The listing builds one solid part. Answer for the finished solid, in the listing's coordinates (mm). Face numbers are marked on the shaded views. A direction names the side the tool comes from. Round coordinates to 2 decimals unless told otherwise and drop trailing zeros. Write each loop counter-clockwise with the first axis right and the second up, starting at its lowest first coordinate (ties: lowest second). Pieces come first, ordered by that corner, then holes.
Item 1: Find the intervals of material crossed by probe 1 along Z at (x, y) = (0, 0.2); probe 2 along Y at (x, z) = (3, -3.5); probe 3 along Y at (x, z) = (2.75, -5), in increasing order.
Item 2: Find section A-A on x = 0. Give the vertices of the cut face in (y, z).
Item 3: A tool of negligible diameter and unlimited length cuts with its end or side. For the marked faces 4, 5 and 6, from which of +Z, -Z, +X, -X, +Y, -Y can it reach the whole face along a straight path? Write none if from no direction.
Item 4: For a pull along Z with two mould halves and no side action, classify the marked faces 1, 2 and 3 as +Z half, -Z half, draft (parallel to the pull), parting line (faces both ways), or undercut.
Item 5: Each of these flat-tipped pins is pushed along its axis until it touches: pin 1 (6 mm diameter, centred on x = -0.5, y = -9, fed in from +Z); pin 2 (3 mm diameter, centred on x = 3, y = -9, fed in from -Z). Where does it stop, or does it pass through?
Item 6: Find section C-C on y = -4.25. Give the vertices of the cut face in (x, z), then the cut area to 3 significant figures.
Item 7: Find section B-B on z = 2.75. Give the vertices of the cut face in (x, y).
```python
from build123d import *

# Parameters (mm, degrees)
EXTRUDE_1_DEPTH              = 3
SKETCH_2_R                   = 5
EXTRUDE_2_DEPTH              = 10
HOLE_WIZARD_M4_1_D           = 6
HOLE_WIZARD_M4_1_CBORE_D     = 10
HOLE_WIZARD_M4_1_CBORE_DEPTH = 4.5


with BuildPart() as part:
    # 草图1 → 凸台-拉伸1 (new, symmetric)
    with BuildSketch(Plane(origin=(0, 0, 0), x_dir=(1, 0, 0), z_dir=(0, 1, 0))):
        Polygon((6.92820323, 0), (3.464101615, 6), (-3.464101615, 6), (-6.92820323, 0), (-3.464101615, -6), (3.464101615, -6), align=None)
    extrude(amount=EXTRUDE_1_DEPTH, both=True)

    # 草图2 → 凸台-拉伸2 (add)
    with BuildSketch(Plane.XZ.offset(3)):
        with Locations(Location((0, 0, 0), (0, 0, 90))):
            Circle(SKETCH_2_R)
    extrude(amount=EXTRUDE_2_DEPTH)

    # M4 六角头螺栓的柱形沉头孔1 (through all)
    with Locations(Plane(origin=(0, 3, 0), x_dir=(1, 0, 0), z_dir=(0, 1, 0))):
        with Locations((0, 0)):
            CounterBoreHole(HOLE_WIZARD_M4_1_D / 2, HOLE_WIZARD_M4_1_CBORE_D / 2, HOLE_WIZARD_M4_1_CBORE_DEPTH)


solid = part.part
```
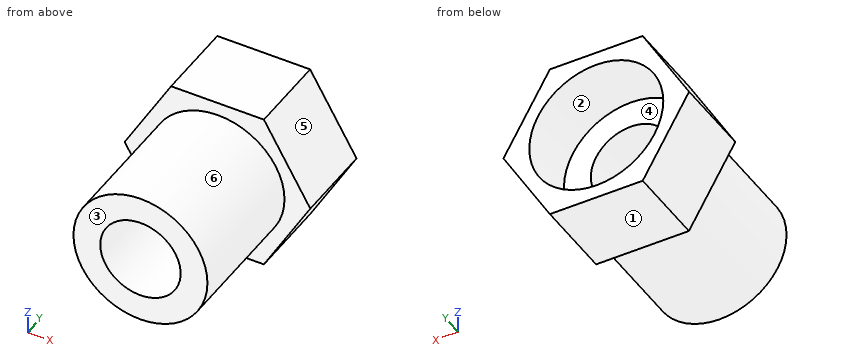
Check values:
1. probe 1: z = -6 to -5, 5 to 6
1. probe 2: y = -13 to -1.5
1. probe 3: y = -3 to 3
2. outline: (-13, -5) - (-3, -5) - (-3, -6) - (3, -6) - (3, -5) - (-1.5, -5) - (-1.5, -3) - (-13, -3) - close; (-13, 3) - (-1.5, 3) - (-1.5, 5) - (3, 5) - (3, 6) - (-3, 6) - (-3, 5) - (-13, 5) - close
3. face 4: +Y
3. face 5: +Z, +X, +Y, -Y
3. face 6: -Y
4. face 1: -Z half
4. face 2: undercut
4. face 3: draft
5. pin 1: stops at z = 5
5. pin 2: stops at z = -4.77
6. outline: circle Ø10 at (0, 0); hole circle Ø6 at (0, 0)
6. area: 50.3 mm2
7. outline: (-5.34, -3) - (-4.18, -3) - (-4.18, -13) - (-1.2, -13) - (-1.2, -1.5) - (-4.18, -1.5) - (-4.18, 3) - (-5.34, 3) - close; (1.2, -13) - (4.18, -13) - (4.18, -3) - (5.34, -3) - (5.34, 3) - (4.18, 3) - (4.18, -1.5) - (1.2, -1.5) - close
